CAD build for the part. Positions are in the model's coordinates, mm. Face numbers are marked on the shaded views. Coordinates: 2 decimals unless noted, no trailing zeros. Write each loop counter-clockwise with the first axis right and the second up, starting at its lowest first coordinate (ties: lowest second). Pieces come first, ordered by that corner, then holes. Notation, with made-up numbers: (-7, -3.5) - (24, -3.5) arc R27 ccw to (24, 23.5) - close; hole circle Ø8 at (59.5, -24). An arc over 180 degrees is marked (long way). Answer in a Markdown table with one row per item. Add a question column.
Q1. Band-saw the part on A-A (x = -112.5). List the corners of the cut face in (y, z), and give its area (3 significant figures).
Q2. Band-saw the part on B-B (y = -208.5). List the corners of the cut face in (x, z).
Q3. Drill centre lines: line 1 along Y through (x, z) = (-445, 1.75); line 2 along Z through (x, y) = (280, -262.5); line 3 along X through (y, z) = (-47, 58). Where is each one in solid material? Low to high. Write a range as from..to.
Q4. Pin check, flat tips, straight feed: pin 1 (1 mm diameter, centred on x = 50.5, z = 61.5, fed in from -Y); pin 2 (2 mm diameter, centred on y = -231.5, z = 17, fed in from -X); pin 3 (5 mm diameter, centred on y = 318.5, z = 78.5, fed in from -X). Stop position of each tip, or through.
Q5. Band-saw the part on C-C (z = 76). List the corners of the cut face in (x, y).
Q6. Two-plate mould, pull along Y, no slides. Class the marked faces 1 and 2: +Y half, -Y half, draft (parallel to the pull), parting line (faces both ways), or undercut.
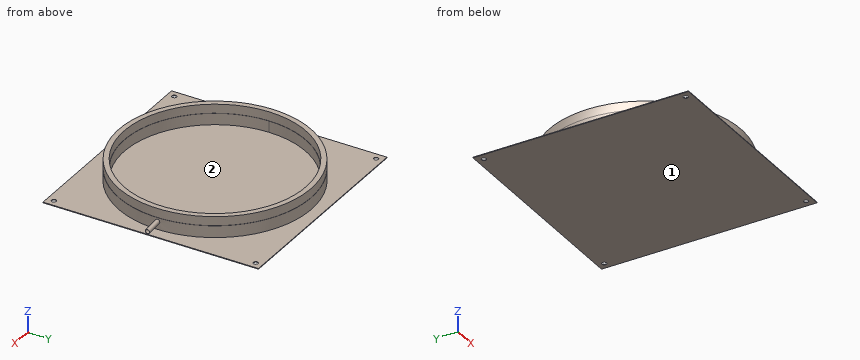
```python
from build123d import *
from build123d import SkipClean  # not in build123d's __all__

# Parameters (mm, degrees)
F0_W     = 10
F0_H     = 3
F2_W     = 950
F2_H     = 950
F2_R     = 10
F3_DEPTH = 3
F6_R     = 9
F7_DEPTH = 120
F8_R     = 400
F9_DEPTH = 200


with BuildPart() as f1:
    # F0 (on Front) → F1 (revolve)
    with BuildSketch(Plane.XZ):
        Polygon((-425, 5), (-400, 5), (-400, 55), (-401, 55), (-401, 95), (-424, 95), (-424, 55), (-425, 55), align=None)
        Polygon((-10, 5), (-400, 5), (-425, 5), (-425, 2), (-10, 2), align=None)
        with Locations((-5, 3.5)):
            Rectangle(F0_W, F0_H)
    revolve(axis=Axis((0, 0, 187.9212413023), (0, 0, -1)))

    # F2 (on Top) → F3 (join)
    with BuildSketch(Plane.XY):
        Rectangle(F2_W, F2_H)
        with Locations((-445, -445)):
            Circle(F2_R, mode=Mode.SUBTRACT)
        with Locations((445, -445)):
            Circle(F2_R, mode=Mode.SUBTRACT)
        with Locations((-445, 445)):
            Circle(F2_R, mode=Mode.SUBTRACT)
        with Locations((445, 445)):
            Circle(F2_R, mode=Mode.SUBTRACT)
    extrude(amount=F3_DEPTH)

    # F4 (on Front) → F5 (revolve)
    with BuildSketch(Plane.XZ):
        Polygon((499.6194698092, 41.5098406888), (400, 50.2254149636), (399.9128442573, 49.2292202655), (499.5323140664, 40.5136459907), align=None)
    revolve(axis=Axis((512.7442754949, 0, 30.3233706049), (0.9961946981, 0, -0.0871557427)))

    # F6 (on face) → F7 (cut)
    with BuildSketch(Plane(origin=(492.2202445211, 0, -43.0636913536), x_dir=(0, 1, 0), z_dir=(0.9961946981, 0, -0.0871557427))):
        with Locations((0, 74.8965891952)):
            Circle(F6_R)
    extrude(amount=-F7_DEPTH, mode=Mode.SUBTRACT)

    # F8 (on face) → F9 (cut)
    with BuildSketch(Plane.XY.offset(5)):
        Circle(F8_R)
    with SkipClean():  # cleaning this boolean's faces spoils the solid; the shape is the same uncleaned
        extrude(amount=F9_DEPTH, mode=Mode.SUBTRACT)


solid = f1.part
```
Checked values:
| question | item | result |
|---|---|---|
| 1 | outline | (-475, 0) - (475, 0) - (475, 3) - (409.84, 3) - (409.84, 55) - (408.8, 55) - (408.8, 95) - (384.9, 95) - (384.9, 55) - (383.85, 55) - (383.85, 5) - (-383.85, 5) - (-383.85, 55) - (-384.9, 55) - (-384.9, 95) - (-408.8, 95) - (-408.8, 55) - (-409.84, 55) - (-409.84, 3) - (-475, 3) - close |
| 1 | area | 9,000 mm² |
| 2 | outline | (-475, 0) - (475, 0) - (475, 3) - (370.34, 3) - (370.34, 55) - (369.19, 55) - (369.19, 95) - (342.53, 95) - (342.53, 55) - (341.36, 55) - (341.36, 5) - (-341.36, 5) - (-341.36, 55) - (-342.53, 55) - (-342.53, 95) - (-369.19, 95) - (-369.19, 55) - (-370.34, 55) - (-370.34, 3) - (-475, 3) - close |
| 3 | line 1 | y = -475..-455, -435..435, 455..475 |
| 3 | line 2 | z = 0..5 |
| 3 | line 3 | x = -421.39..-398.24, 398.24..421.39 |
| 4 | pin 1 | stops at y = -421.04 |
| 4 | pin 2 | stops at x = -357.06 |
| 4 | pin 3 | stops at x = -282.7 |
| 5 | outline | circle Ø848 at (0, 0); hole circle Ø802 at (0, 0) |
| 6 | face 1 | draft |
| 6 | face 2 | undercut |
